Check sheet for the modelled part. Datum: model origin and axes. Units: mm. A direction names the side the tool comes from. Round coordinates to 2 decimals unless told otherwise and drop trailing zeros. Write each loop counter-clockwise with the first axis right and the second up, starting at its lowest first coordinate (ties: lowest second). Pieces come first, ordered by that corner, then holes. Notation, with made-up numbers: (-35.75, 43) -> (-4.75, 43) arc R4 ccw to (-4.75, 50) -> close; hole circle Ø11 at (35, -35). An arc over 180 degrees is marked (long way). Write item = value, one per line.
from build123d import *

# Parameters (mm, degrees)
F0_W     = 804
F0_H     = 775
F0_W_2   = 752.827108
F0_H_2   = 230.544425
F0_W_3   = 751.404017
F0_H_3   = 123.810884
F0_H_4   = 118.118427
F0_W_4   = 754.250229
F0_H_5   = 119.541556
F1_DEPTH = 483


with BuildPart() as f1:
    # F0 (on Front) → F1 (new body)
    with BuildSketch(Plane.XZ):
        Rectangle(F0_W, F0_H)
        with Locations((-1.859218, -230.949025)):
            Rectangle(F0_W_2, F0_H_2, mode=Mode.SUBTRACT)
        with Locations((-1.147672, -22.462869)):
            Rectangle(F0_W_3, F0_H_3, mode=Mode.SUBTRACT)
        with Locations((-1.859218, 138.34897)):
            Rectangle(F0_W_2, F0_H_4, mode=Mode.SUBTRACT)
        with Locations((-1.147658, 291.33369)):
            Rectangle(F0_W_4, F0_H_5, mode=Mode.SUBTRACT)
    extrude(amount=F1_DEPTH)


solid = f1.part
(1) Access from +Z, -Z, +X, -X, +Y, -Y to the whole of each face (thin tool, end or side, straight path). Record for faces 1 (the flat face through (-32, 0, 59)), 2 (the flat face through (374.554, -238, 138)).
Worked answers:
face_1 = +Z, -Z, +X, -X, +Y
face_2 = +Y, -Y
(2) Sectioned sample at B-B on y = -353.5. Enter the section's corners in (x, z), then the cut area to 3 significant figures.
Worked answers:
outline = (-402, -387.5) -> (402, -387.5) -> (402, 387.5) -> (-402, 387.5) -> close; hole (-378.27, -346.22) -> (374.55, -346.22) -> (374.55, -115.68) -> (-378.27, -115.68) -> close; hole (-378.27, 79.29) -> (374.55, 79.29) -> (374.55, 197.41) -> (-378.27, 197.41) -> close; hole (-378.27, 231.56) -> (375.98, 231.56) -> (375.98, 351.1) -> (-378.27, 351.1) -> close; hole (-376.85, -84.37) -> (374.55, -84.37) -> (374.55, 39.44) -> (-376.85, 39.44) -> close
area = 177,000 mm²
(3) Release check for a two-part mould opening along Z. For faces 3 (the flat face through (-402, -238, -5)), 4 (the flat face through (-7, -238, -115.677)), 5 (the flat face through (-6, -238, -387.5)) record: pulls with the +Z half, pulls with the -Z half, needs draft (parallel to the pull), parting line crosses it, or undercut.
Worked answers:
face_3 = needs draft
face_4 = undercut
face_5 = pulls with the -Z half
(4) Sectioned sample at A-A on z = 174.5. Enter the section's corners in (x, y), then the cut area to 3 significant figures.
Worked answers:
outline = (-402, -483) -> (-378.27, -483) -> (-378.27, 0) -> (-402, 0) -> close; (374.55, -483) -> (402, -483) -> (402, 0) -> (374.55, 0) -> close
area = 24,700 mm²
(5) Sectioned sample at C-C on x = -164. Enter the section's corners in (y, z), then the cut area to 3 significant figures.
Worked answers:
outline = (-483, -387.5) -> (0, -387.5) -> (0, -346.22) -> (-483, -346.22) -> close; (-483, -115.68) -> (0, -115.68) -> (0, -84.37) -> (-483, -84.37) -> close; (-483, 39.44) -> (0, 39.44) -> (0, 79.29) -> (-483, 79.29) -> close; (-483, 197.41) -> (0, 197.41) -> (0, 231.56) -> (-483, 231.56) -> close; (-483, 351.1) -> (0, 351.1) -> (0, 387.5) -> (-483, 387.5) -> close
area = 88,400 mm²
(6) Material ranges on L1, parallel to Z at x = 351, y = -285; L2, parallel to X at y = -362, z = 95.5; L3, parallel to X at y = -286, z = 253.5, recorded low to high. Write a range as [from, to].
Worked answers:
L1 = [-387.5, -346.22], [-115.68, -84.37], [39.44, 79.29], [197.41, 231.56], [351.1, 387.5]
L2 = [-402, -378.27], [374.55, 402]
L3 = [-402, -378.27], [375.98, 402]
(7) Sectioned sample at D-D on z = -4. Enter the section's corners in (x, y).
Worked answers:
outline = (-402, -483) -> (-376.85, -483) -> (-376.85, 0) -> (-402, 0) -> close; (374.55, -483) -> (402, -483) -> (402, 0) -> (374.55, 0) -> close
